Could you check a few things on this drawing? It's one solid part, dimensions in mm from its lowest x, y, z. Give positions to 0.01 mm unless a question says otherwise; leave off trailing zeros. Write each loop counter-clockwise with the first axis right and the second up, starting at its lowest first coordinate (ties: lowest second). Pieces come first, ordered by that corner, then holes. Notation, with made-up numbers: (-18, 58.5) - (-11, 58.5) arc R19 ccw to (-11, 94.5) - close; hole circle Ø11 at (33, 63.25). An arc over 180 degrees is marked (long way). One line per item, written item: value. Start each with the question number.
1) Imagine slicing it at D-D on z = 49. Write out the boundary of the cut face in (x, y).
2) Imagine slicing it at B-B on y = 25. Write out the boundary of the cut face in (x, z).
3) Please list where these lines run through material, in increasing order: L1, parallel to X at y = 23.5, z = 41.5; L2, parallel to Z at x = 15, y = 24; L3, parallel to Y at x = 23.5, z = 53. Write a range as [from, to].
4) I'm going to push flat-ended pins straight in: P1, Ø5, axis at x = 30.5, y = 34, coming from the +Z side; P2, Ø5, axis at y = 22.5, z = 49.5, coming from the +X side; P3, Ø5, axis at y = 16.5, z = 48.5, coming from the -X side. Where does each tip first touch, or does it pass through?
5) We'd pull the mould along X, two halves only. Please class the marked faces 1, 2, 3 and 4: +X half, -X half, draft (parallel to the pull), parting line (faces both ways), or undercut.
6) Imagine slicing it at A-A on z = 40. Write out the boundary of the cut face in (x, y), plus the area to 3 significant figures.
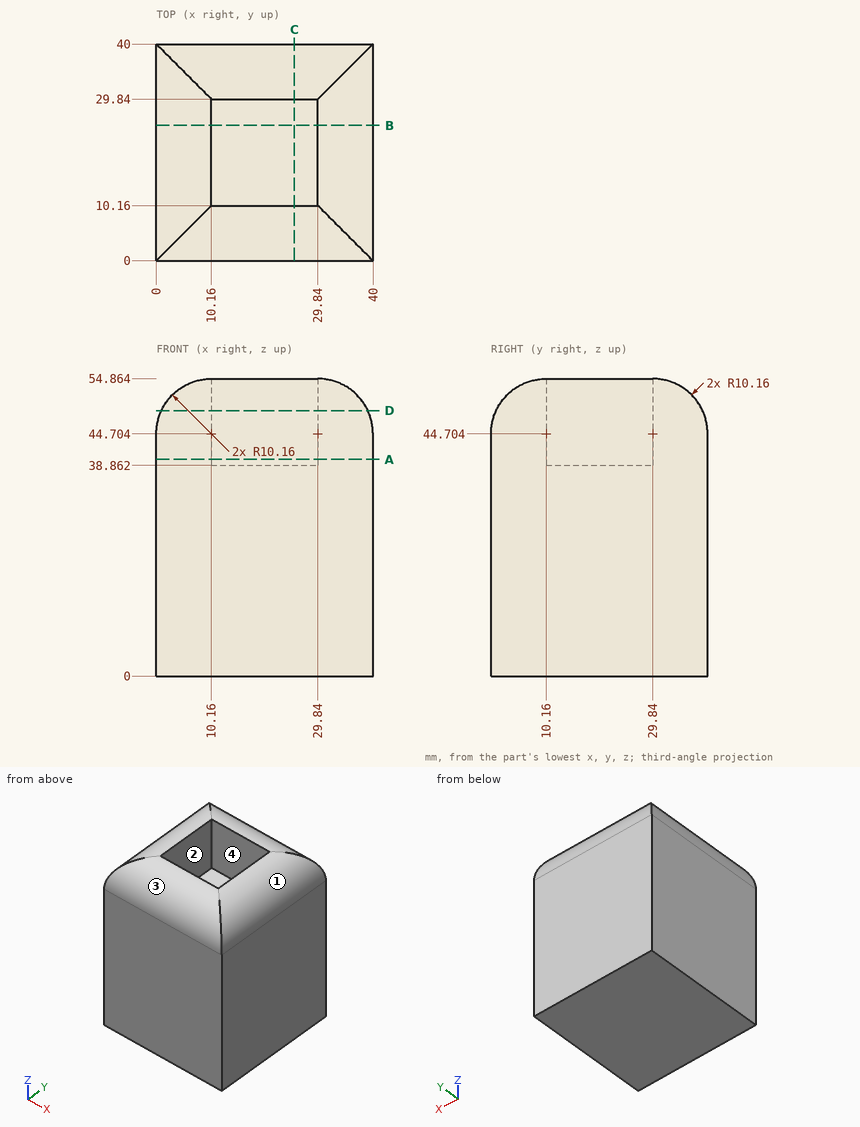
Numbers:
1. outline: (0.95, 0.95) - (39.05, 0.95) - (39.05, 39.05) - (0.95, 39.05) - close; hole (10.16, 10.16) - (29.84, 10.16) - (29.84, 29.84) - (10.16, 29.84) - close
2. outline: (0, 0) - (40, 0) - (40, 44.7) arc R10.16 ccw to (29.84, 54.86) - (29.84, 38.86) - (10.16, 38.86) - (10.16, 54.86) arc R10.16 ccw to (0, 44.7) - close
3. L1: [0, 10.16], [29.84, 40]
3. L2: [0, 38.86]
3. L3: [4.29, 10.16], [29.84, 35.71]
4. P1: z = 54.73
4. P2: x = 39.74
4. P3: x = 0.08
5. face 1: +X half
5. face 2: undercut
5. face 3: draft
5. face 4: undercut
6. outline: (0, 0) - (40, 0) - (40, 40) - (0, 40) - close; hole (10.16, 10.16) - (29.84, 10.16) - (29.84, 29.84) - (10.16, 29.84) - close
6. area: 1,210 mm^2
